from build123d import *

# Parameters (mm, degrees)
SKETCH_1_R          = 11
SKETCH_1_R_2        = 4.15
EXTRUDE_1_DEPTH     = 2
EXTRUDE_START       = 5
SKETCH_1_3_R        = 5.65
SKETCH_1_3_R_2      = 4.15
EXTRUDE_2_DEPTH     = 5
CUT_EXTRUDE_1_DEPTH = 4


with BuildPart() as part:
    # Sketch 1 → Extrude 1 (new body)
    with BuildSketch(Plane(origin=(0, 0, 0), x_dir=(1, 0, 0), z_dir=(0, 1, 0))):
        with Locations(Location((0, 0, 0), (0, 0, 270))):
            Circle(SKETCH_1_R)
        with Locations(Location((0, 0, 0), (0, 0, 270))):
            Circle(SKETCH_1_R_2, mode=Mode.SUBTRACT)
    extrude(amount=-EXTRUDE_1_DEPTH)

    # Sketch 1_3 → Extrude 2 (add)
    with BuildSketch(Plane(origin=(0, 0, 0), x_dir=(1, 0, 0), z_dir=(0, 1, 0)).offset(EXTRUDE_START)):
        with Locations(Location((0, 0, 0), (0, 0, 270))):
            Circle(SKETCH_1_3_R)
        with Locations(Location((0, 0, 0), (0, 0, 270))):
            Circle(SKETCH_1_3_R_2, mode=Mode.SUBTRACT)
    extrude(amount=-EXTRUDE_2_DEPTH)

    # Sketch 2 → Cut-Extrude 1 (cut)
    with BuildSketch(Plane(origin=(0, 5, 0), x_dir=(1, 0, 0), z_dir=(0, 1, 0))):
        with BuildLine():
            Line((1.95, 5.302829433), (1.95, 3.663331817))
            ThreePointArc((1.95, 3.663331817), (4.15, 0), (1.95, -3.663331817))
            Line((1.95, -3.663331817), (1.95, -5.302829433))
            ThreePointArc((1.95, -5.302829433), (5.65, 0), (1.95, 5.302829433))
        make_face()
        with BuildLine():
            Line((-1.95, 5.302829433), (-1.95, 3.663331817))
            ThreePointArc((-1.95, 3.663331817), (-4.15, 0), (-1.95, -3.663331817))
            Line((-1.95, -3.663331817), (-1.95, -5.302829433))
            ThreePointArc((-1.95, -5.302829433), (-5.65, 0), (-1.95, 5.302829433))
        make_face()
    extrude(amount=-CUT_EXTRUDE_1_DEPTH, mode=Mode.SUBTRACT)


solid = part.part
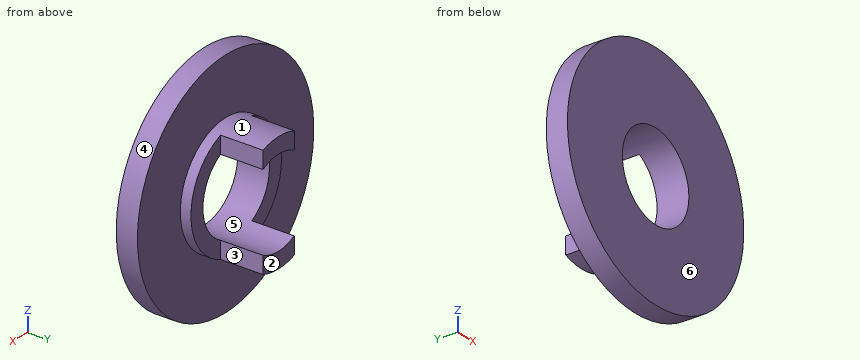
CAD build for the part. Positions are in the model's coordinates, mm. Face numbers are marked on the shaded views. A direction names the side the tool comes from. Coordinates: 2 decimals unless noted, no trailing zeros. Write each loop counter-clockwise with the first axis right and the second up, starting at its lowest first coordinate (ties: lowest second). Pieces come first, ordered by that corner, then holes. Notation, with made-up numbers: M 89.5,67.5 L 104.5,67.5 A21 cw 104.5,96.5 Z; hole C 10,84 d7. An arc over 180 degrees is marked long. Return JSON: item names as keys, results as strings.
Item 1: Slice it at C-C, the plane y = -1.5. Write the cut outline in (x, z), and give its area (3 significant figures).
Findings below:
{"outline": "C 0,0 d22; hole C 0,0 d8.3", "area": "326 mm2"}
Item 2: Which spindle directions (+Z, -Z, +X, -X, +Y, -Y) get a long thin tool onto all of the face, cutting with end or side? Do the marked faces 1, 2 and 3. Say none if no direction does.
Findings below:
{"face 1": "+Y", "face 2": "+Z, -Z, +X, -X, +Y", "face 3": "+Z, -Z, +X, +Y"}
Item 3: Slice it at B-B, the plane z = 0. Write the cut outline in (x, y).
Findings below:
{"outline": "M -11,-2 L -4.15,-2 L -4.15,1 L -5.65,1 L -5.65,0 L -11,0 Z; M 4.15,-2 L 11,-2 L 11,0 L 5.65,0 L 5.65,1 L 4.15,1 Z"}
Item 4: Drop flat-ended pins along their axis: pin 1 Ø0.5 at (y, z) = (3.5, 4) entering from +X; pin 2 Ø0.8 at (y, z) = (3, 5) entering from -X; pin 3 Ø11 at (x, z) = (-1, -2) entering from +Y; pin 4 Ø1 at (y, z) = (-1, 2) entering from -X. Give the stop position or say it passes through.
Findings below:
{"pin 1": "stops at x = 1.95", "pin 2": "stops at x = -1.95", "pin 3": "stops at y = 5", "pin 4": "stops at x = -10.9"}
Item 5: Slice it at D-D, the plane z = 8.5. Write the cut outline in (x, y).
Findings below:
{"outline": "M -6.98,-2 L 6.98,-2 L 6.98,0 L -6.98,0 Z"}
Item 6: Two-plate mould, pull along Z, no slides. Class the marked faces 4, 5 and 6: +Z half, -Z half, draft (parallel to the pull), parting line (faces both ways), or undercut.
Findings below:
{"face 4": "parting line", "face 5": "undercut", "face 6": "draft"}
Item 7: Probe line 1 (Z direction, x = 0, y = 0.75); line 2 (Y direction, x = -2.75, z = -4.75). List the from-to ranges inside material, lowest first. Write a range as from..to.
Findings below:
{"line 1": "z = -5.65..-4.15, 4.15..5.65", "line 2": "y = -2..1"}
Item 8: Slice it at A-A, the plane x = 0. Write the cut outline in (y, z), and give its area (3 significant figures).
Findings below:
{"outline": "M -2,-11 L 0,-11 L 0,-5.65 L 5,-5.65 L 5,-4.15 L -2,-4.15 Z; M -2,4.15 L 5,4.15 L 5,5.65 L 0,5.65 L 0,11 L -2,11 Z", "area": "42.4 mm2"}
